Read the model definition and answer for the solid it produces. Units are mm, in the model's axes. Face numbers are marked on the shaded views. A direction names the side the tool comes from. Give positions to 0.01 mm unless a question says otherwise; leave off trailing zeros. Order: outer loops, then holes, each group sorted by start corner. A loop starts at its lowest first (then second) coordinate and runs counter-clockwise, first axis right, second up. Notation, with made-up numbers: (-5, -15.5) - (4, -15.5) arc R21 ccw to (4, 12.5) - close; hole circle Ø8 at (-37.75, -24.5). An arc over 180 degrees is marked (long way). Write each question's results on one line, items separated by ' | '. Start each with the question number.
Q1. Find section B-B on x = -25. Give the vertices of the cut face in (y, z), and give its area (3 significant figures).
Q2. Find section A-A on y = 65.5. Give the vertices of the cut face in (x, z).
Q3. Find section C-C on x = 6.65. Give the vertices of the cut face in (y, z), and give its area (3 significant figures).
Q4. A tool of negligible diameter and unlimited length cuts with its end or side. For the marked faces 1, 2 and 3, from which of +Z, -Z, +X, -X, +Y, -Y can it reach the whole face along a straight path? Write none if from no direction.
Q5. Find the intervals of material crossed by line 1 along X through (y, z) = (62.85, -18.1); line 2 along Y through (x, z) = (-11.5, -17); line 3 along Z through (x, y) = (-4, -10.9), in increasing order. Write a range as from..to.
Q6. Find section D-D on y = 28. Give the vertices of the cut face in (x, z).
Q7. Flat-ended cylindrical pins translate along their axes: P1, Ø5.5, axis at x = 27.1, z = -18.1, coming from the +Y side; P2, Ø1.8, axis at x = -58.9, z = 1, coming from the +Y side; P3, Ø1, axis at y = 21, z = -12.5, coming from the -X side. Find the tip coordinate at first contact, or state that the pin passes through.
Q8. For a pull along Y with two mould halves and no side action, classify the marked faces 4, 5 and 6 as +Y half, -Y half, draft (parallel to the pull), parting line (faces both ways), or undercut.
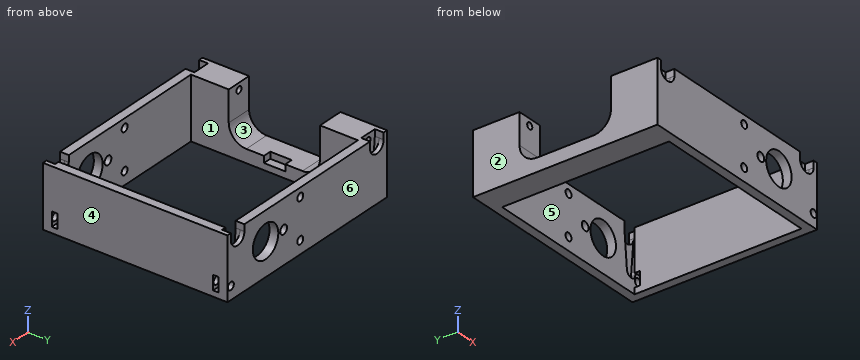
from build123d import *

# Parameters (mm, degrees)
SALIENTE_EXTRUIR1_DEPTH      = 4
SALIENTE_EXTRUIR1_DEPTH_BACK = 24
CROQUIS1_W                   = 94
CROQUIS1_H                   = 84
CROQUIS1_W_2                 = 78
CROQUIS1_H_2                 = 76
CROQUIS10_R                  = 1.5
CORTAR_EXTRUIR6_DEPTH        = 109.830188826
CORTAR_EXTRUIR1_DEPTH        = 2
CORTAR_EXTRUIR5_DEPTH        = 2
CORTAR_EXTRUIR2_REACH        = 122.073
CROQUIS12_R                  = 7.5
CROQUIS12_R_2                = 1.75
CROQUIS12_R_3                = 2
CORTAR_EXTRUIR7_DEPTH        = 10
CROQUIS17_W                  = 4
CROQUIS17_H                  = 9.7
CORTAR_EXTRUIR10_DEPTH       = 3
CORTAR_EXTRUIR11_DEPTH       = 2.5
SIMETR_A2_COPY_1_DEPTH       = 2
SIMETR_A2_COPY_2_DEPTH       = 2


with BuildPart() as part:
    # Croquis1 → Saliente-Extruir1 (new, two sides: drawn at the far end of the back side and taken through both)
    with BuildSketch(Plane.XY.offset(-SALIENTE_EXTRUIR1_DEPTH_BACK)):
        with Locations((-17.9, 28.75)):
            Rectangle(CROQUIS1_W, CROQUIS1_H)
        with Locations((-13.9, 28.75)):
            Rectangle(CROQUIS1_W_2, CROQUIS1_H_2, mode=Mode.SUBTRACT)
    extrude(amount=SALIENTE_EXTRUIR1_DEPTH + SALIENTE_EXTRUIR1_DEPTH_BACK)

    # Croquis10 → Cortar-Extruir6 (cut, through all)
    with BuildSketch(Plane(origin=(0, 70.75, 0), x_dir=(1, 0, 0), z_dir=(0, 1, 0))):
        with Locations(Location((-58.9, -1, 0), (0, 0, 180))):
            Circle(CROQUIS10_R)
    extrude(amount=-CORTAR_EXTRUIR6_DEPTH, mode=Mode.SUBTRACT)

    # Croquis2 → Cortar-Extruir1 (cut)
    with BuildSketch(Plane(origin=(0, -13.25, 0), x_dir=(-1, 0, 0), z_dir=(0, -1, 0))):
        with BuildLine():
            Line((54.9, -1), (54.9, -4))
            Line((54.9, -4), (62.9, -4))
            Line((62.9, -4), (62.9, -1))
            ThreePointArc((62.9, -1), (58.9, 3), (54.9, -1))
        make_face()
    cortar_extruir1 = extrude(amount=-CORTAR_EXTRUIR1_DEPTH, mode=Mode.SUBTRACT)

    # Croquis9 → Cortar-Extruir5 (cut)
    with BuildSketch(Plane(origin=(0, -9.25, 0), x_dir=(1, 0, 0), z_dir=(0, 1, 0))):
        with BuildLine():
            Line((-61.389870926, 15.724817194), (-62.9, -1))
            Line((-62.9, -1), (-62.9, -4))
            Line((-62.9, -4), (-54.9, -4))
            Line((-54.9, -4), (-54.9, -1))
            Line((-54.9, -1), (-56.410129074, 15.724817194))
            ThreePointArc((-56.410129074, 15.724817194), (-58.9, 18), (-61.389870926, 15.724817194))
        make_face()
    cortar_extruir5 = extrude(amount=-CORTAR_EXTRUIR5_DEPTH, mode=Mode.SUBTRACT)

    # Croquis5 → Cortar-Extruir2 (cut, up to next)
    with BuildSketch(Plane.ZY.offset(64.9), mode=Mode.PRIVATE) as cortar_extruir2_sk1:
        with BuildLine():
            Line((-18, 41.55), (-18, 15.95))
            ThreePointArc((-18, 15.95), (-15.656854249, 10.293145751), (-10, 7.95))
            Line((-10, 7.95), (4, 7.95))
            Line((4, 7.95), (4, 49.55))
            Line((4, 49.55), (-10, 49.55))
            ThreePointArc((-10, 49.55), (-15.656854249, 47.206854249), (-18, 41.55))
        make_face()
    cortar_extruir2_tool1 = extrude(cortar_extruir2_sk1.sketch, amount=-CORTAR_EXTRUIR2_REACH, mode=Mode.PRIVATE) & part.part
    add(cortar_extruir2_tool1.solids().sort_by_distance((-64.9, 28.75, -6.714921))[0], mode=Mode.SUBTRACT)

    # Croquis12 → Cortar-Extruir7 (cut)
    with BuildSketch(Plane.XZ.offset(13.25)):
        with Locations((6.65, -9.05)):
            Circle(CROQUIS12_R)
        with Locations((-13.8, 0)):
            Circle(CROQUIS12_R_2)
        with Locations((-13.8, -18.1)):
            Circle(CROQUIS12_R_2)
        with Locations((-4, -9.05)):
            Circle(CROQUIS12_R_3)
        with Locations(Location((27.1, -18.1, 0), (0, 0, 180))):
            Circle(CROQUIS12_R_2)
    cortar_extruir7 = extrude(amount=-CORTAR_EXTRUIR7_DEPTH, mode=Mode.SUBTRACT)

    # Croquis17 → Cortar-Extruir10 (cut)
    with BuildSketch(Plane.XY.offset(-18)):
        with Locations((-54.655566502, 28.846197779)):
            Rectangle(CROQUIS17_W, CROQUIS17_H)
    extrude(amount=-CORTAR_EXTRUIR10_DEPTH, mode=Mode.SUBTRACT)

    # Croquis20 → Cortar-Extruir11 (cut)
    with BuildSketch(Plane(origin=(0, -9.25, 0), x_dir=(-1, 0, 0), z_dir=(0, -1, 0))):
        Polygon((-29.1, 14.85), (-27.1, 14.85), (-25.223611625, 14.85), (-24.285417438, 16.475), (-23.34722325, 18.1), (-24.285417438, 19.725), (-25.223611625, 21.35), (-27.1, 21.35), (-29.1, 21.35), align=None)
    cortar_extruir11 = extrude(amount=-CORTAR_EXTRUIR11_DEPTH, mode=Mode.SUBTRACT)

    # Simetr_a3: Cortar-Extruir1, Cortar-Extruir5 across plane
    add(cortar_extruir1.mirror(Plane.ZY.offset(17.9)), mode=Mode.SUBTRACT)
    add(cortar_extruir5.mirror(Plane.ZY.offset(17.9)), mode=Mode.SUBTRACT)

    # Simetr_a2: Cortar-Extruir1, Cortar-Extruir5, Cortar-Extruir7, Cortar-Extruir11 across plane
    add(cortar_extruir1.mirror(Plane(origin=(0, 28.75, 0), x_dir=(0, 0, 1), z_dir=(0, -1, 0))), mode=Mode.SUBTRACT)
    add(cortar_extruir5.mirror(Plane(origin=(0, 28.75, 0), x_dir=(0, 0, 1), z_dir=(0, -1, 0))), mode=Mode.SUBTRACT)
    add(cortar_extruir7.mirror(Plane(origin=(0, 28.75, 0), x_dir=(0, 0, 1), z_dir=(0, -1, 0))), mode=Mode.SUBTRACT)
    add(cortar_extruir11.mirror(Plane(origin=(0, 28.75, 0), x_dir=(0, 0, 1), z_dir=(0, -1, 0))), mode=Mode.SUBTRACT)

    # Simetr_a2 copy 1 sketch → Simetr_a2 copy 1 (cut)
    with BuildSketch(Plane(origin=(-35.8, 70.75, 0), x_dir=(1, 0, 0), z_dir=(0, 1, 0))):
        with BuildLine():
            Line((54.9, -1), (54.9, -4))
            Line((54.9, -4), (62.9, -4))
            Line((62.9, -4), (62.9, -1))
            ThreePointArc((62.9, -1), (58.9, 3), (54.9, -1))
        make_face()
    extrude(amount=-SIMETR_A2_COPY_1_DEPTH, mode=Mode.SUBTRACT)

    # Simetr_a2 copy 2 sketch → Simetr_a2 copy 2 (cut)
    with BuildSketch(Plane(origin=(-35.8, 66.75, 0), x_dir=(-1, 0, 0), z_dir=(0, -1, 0))):
        with BuildLine():
            Line((-61.389870926, 15.724817194), (-62.9, -1))
            Line((-62.9, -1), (-62.9, -4))
            Line((-62.9, -4), (-54.9, -4))
            Line((-54.9, -4), (-54.9, -1))
            Line((-54.9, -1), (-56.410129074, 15.724817194))
            ThreePointArc((-56.410129074, 15.724817194), (-58.9, 18), (-61.389870926, 15.724817194))
        make_face()
    extrude(amount=-SIMETR_A2_COPY_2_DEPTH, mode=Mode.SUBTRACT)


solid = part.part
Working result:
1) outline: (-13.25, -24) - (-9.25, -24) - (-9.25, 4) - (-13.25, 4) - close; (66.75, -24) - (70.75, -24) - (70.75, 4) - (66.75, 4) - close | area: 224 mm²
2) outline: (-64.9, -24) - (-52.9, -24) - (-52.9, 4) - (-64.9, 4) - close; (25.1, -24) - (29.1, -24) - (29.1, -21.35) - (25.22, -21.35) - (25.1, -21.14) - close; (25.1, -15.06) - (25.22, -14.85) - (29.1, -14.85) - (29.1, 4) - (25.1, 4) - close; hole circle Ø3 at (-58.9, 1)
3) outline: (-13.25, -24) - (-9.25, -24) - (-9.25, -16.55) - (-13.25, -16.55) - close; (-13.25, -1.55) - (-9.25, -1.55) - (-9.25, 4) - (-13.25, 4) - close; (66.75, -24) - (70.75, -24) - (70.75, -16.55) - (66.75, -16.55) - close; (66.75, -1.55) - (70.75, -1.55) - (70.75, 4) - (66.75, 4) - close | area: 104 mm²
4) face 1: +Z, -Z | face 2: +Z, -Z, -X, +Y, -Y | face 3: +Z, -X
5) line 1: -64.9..-52.9, 25.1..25.35, 28.85..29.1 | line 2: -13.25..-9.25, 66.75..70.75 | line 3: -24..-11.05, -7.05..4
6) outline: (-64.9, -24) - (-52.9, -24) - (-52.9, -21) - (-56.66, -21) - (-56.66, -18) - (-64.9, -18) - close; (25.1, -24) - (29.1, -24) - (29.1, 4) - (25.1, 4) - close
7) P1: y = 70.75 | P2: through | P3: x = 25.1
8) face 4: draft | face 5: undercut | face 6: +Y half
